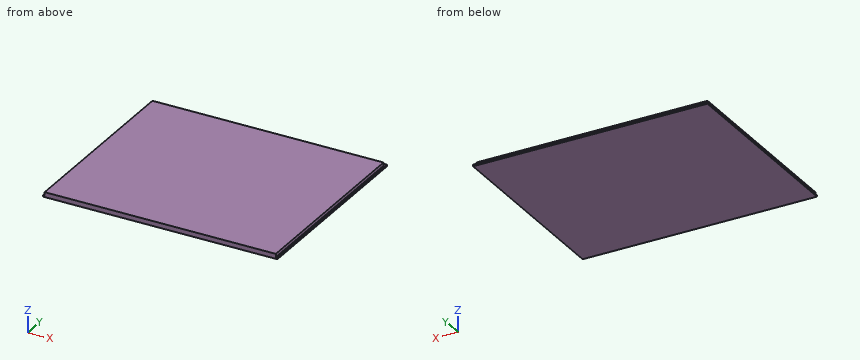
```python
from build123d import *

# Parameters (mm, degrees)
F0_W     = 914.4
F0_H     = 762
F1_DEPTH = 19.05
F2_W     = 6.35
F2_H     = 12.7
F3_DEPTH = 762.001
F4_W     = 12.7
F4_H     = 12.7
F5_DEPTH = 914.401


with BuildPart() as f1:
    # F0 (on Top) → F1 (new body)
    with BuildSketch(Plane.XY):
        with Locations((457.2, 381)):
            Rectangle(F0_W, F0_H)
    extrude(amount=F1_DEPTH)

    # F2 (on face) → F3 (cut, through all)
    with BuildSketch(Plane.XZ):
        with Locations((3.175, 12.7)):
            Rectangle(F2_W, F2_H)
        with Locations((911.225, 12.7)):
            Rectangle(F2_W, F2_H)
    extrude(amount=-F3_DEPTH, mode=Mode.SUBTRACT)

    # F4 (on face) → F5 (cut, through all)
    with BuildSketch(Plane.YZ.offset(914.4)):
        with Locations((755.65, 12.7)):
            Rectangle(F4_W, F4_H)
    extrude(amount=-F5_DEPTH, mode=Mode.SUBTRACT)


solid = f1.part
```
Geometry: final body of the model. Coordinates: model frame, mm. Coordinates: 2 decimals unless noted, no trailing zeros. Order: outer loops, then holes, each group sorted by start corner. A loop starts at its lowest first (then second) coordinate and runs counter-clockwise, first axis right, second up.
Item 1: Contact query for flat-ended pins moving along their axis: P1, Ø4, axis at y = 540, z = 15.5, coming from the -X side; P2, Ø8, axis at x = 245, z = 11, coming from the -Y side; P3, Ø4, axis at x = 333.5, z = 14, coming from the +Y side. Output: stop coordinate, or through.
Answer:
P1: stops at x = 6.35
P2: stops at y = 0
P3: stops at y = 749.3
Item 2: Material intervals for line 1 along Y through (x, z) = (124, 10.5); line 2 along X through (y, z) = (320.5, 6.5), sorted ascending.
Answer:
line 1: y = 0 to 749.3
line 2: x = 6.35 to 908.05
Item 3: Section query A-A (z = 12.75). Output: boundary loops of the cut face in (x, y).
Answer:
outline: (6.35, 0) - (908.05, 0) - (908.05, 749.3) - (6.35, 749.3) - close
